Here's the drawing with two shaded views (mm, measured from the low corner). I have some questions. Coordinates: 2 decimals unless noted, no trailing zeros. Write each loop counter-clockwise with the first axis right and the second up, starting at its lowest first coordinate (ties: lowest second). Pieces come first, ordered by that corner, then holes. Notation, with made-up numbers: (71, -9.75) -> (109, -9.75) arc R22 cw to (109, 22.25) -> close; hole circle Ø10 at (52, 62.5). An arc over 180 degrees is marked (long way). Use a Markdown table: item, result. Add a question column.
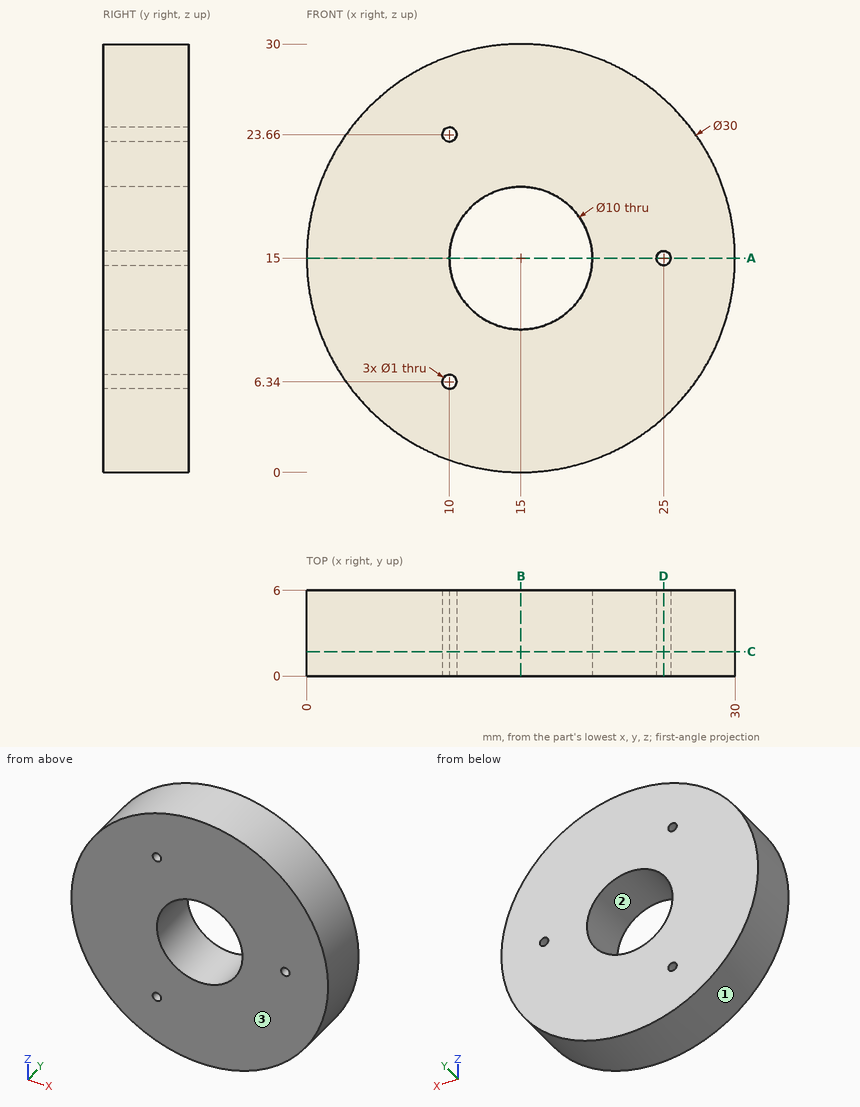
Q1. Will these pins go through, and if not, where does the flat tip stop? pin 1 (6 mm diameter, centred on x = 15, z = 15, fed in from -Y); pin 2 (3 mm diameter, centred on y = 5, z = 24.5, fed in from -X); pin 3 (1 mm diameter, centred on y = 2.5, z = 24, fed in from +X).
Q2. Suppose I cut it at D-D, the plane x = 25. Write out the boundary of the cut face in (y, z).
Q3. Suppose I cut it at B-B, the plane x = 15. Write out the boundary of the cut face in (y, z), and give its area (3 significant figures).
Q4. Thinking about a two-plate mould opening in Z: for the marked faces 1, 2 and 3, which applies, released by +Z, released by -Z, zero draft, split by the parting line, or undercut?
Q5. Suppose I cut it at A-A, the plane z = 15. Write out the boundary of the cut face in (x, y).
Q6. Suppose I cut it at C-C, the plane y = 1.7. Write out the boundary of the cut face in (x, z).
Q7. Please list where these lines run through material, in increasing order: line 1 (Z direction, x = 15, y = 4.3); line 2 (X direction, y = 4.65, z = 16.5) (1 decimal); line 3 (X direction, y = 2.4, z = 6).
Answer key:
| question | item | result |
|---|---|---|
| 1 | pin 1 | passes through |
| 1 | pin 2 | stops at x = 2.31 |
| 1 | pin 3 | stops at x = 27.36 |
| 2 | outline | (0, 3.82) -> (6, 3.82) -> (6, 14.5) -> (0, 14.5) -> close; (0, 15.5) -> (6, 15.5) -> (6, 26.18) -> (0, 26.18) -> close |
| 3 | outline | (0, 0) -> (6, 0) -> (6, 10) -> (0, 10) -> close; (0, 20) -> (6, 20) -> (6, 30) -> (0, 30) -> close |
| 3 | area | 120 mm^2 |
| 4 | face 1 | split by the parting line |
| 4 | face 2 | undercut |
| 4 | face 3 | zero draft |
| 5 | outline | (0, 0) -> (10, 0) -> (10, 6) -> (0, 6) -> close; (20, 0) -> (24.5, 0) -> (24.5, 6) -> (20, 6) -> close; (25.5, 0) -> (30, 0) -> (30, 6) -> (25.5, 6) -> close |
| 6 | outline | circle Ø30 at (15, 15); hole circle Ø1 at (10, 6.34); hole circle Ø1 at (10, 23.66); hole circle Ø10 at (15, 15); hole circle Ø1 at (25, 15) |
| 7 | line 1 | z = 0 to 10, 20 to 30 |
| 7 | line 2 | x = 0.1 to 10.2, 19.8 to 29.9 |
| 7 | line 3 | x = 3 to 9.63, 10.37 to 27 |
